Could you check a few things on this model? Use its own coordinates, in mm. A direction names the side the tool comes from. Coordinates: 2 decimals unless noted, no trailing zeros. Loops run counter-clockwise (first coordinate to the right, second up) from the corner with the lowest first, then second, coordinate; pieces in that order, holes last. Notation, with made-up numbers: (41.25, -9) - (50.25, -9) arc R14 ccw to (50.25, 15) - close; hole circle Ø2 at (4, 9.5). An arc over 180 degrees is marked (long way). Put each result on its own line as item: value. Start each with the question number.
```python
from build123d import *

# Parameters (mm, degrees)
F1_DEPTH    = 25
F2_SIZE2    = 24.99999
F2_SIZE     = 77.78174
F4_DEPTH    = 130
F5_W        = 126.5929291126
F5_H        = 5
F6_DEPTH    = 25
F7_T1_DEPTH = 126.5929291126
F9_DEPTH    = 15


# Not quite as in the source:
# - a fillet or chamfer that OpenCascade refuses, or shapes differently, is made with other operations: its cross-section is extruded or revolved along the edge and cut away or added
# - a fillet or chamfer is up to 0.001 mm smaller than in the source, because OpenCascade refuses the exact size


with BuildPart() as f1:
    # F0 (on Top) → F1 (new body)
    with BuildSketch(Plane.XY):
        Polygon((55, 55), (-55, 55), (-55, -55), align=None)
    extrude(amount=F1_DEPTH)

    # F2 (size 77.78175 and 25 in the source; OpenCascade refuses exactly that, so slightly less here)
    f2_edges = [f1.edges().sort_by_distance(p)[0] for p in [
        (0, 0, 25),
    ]]
    f2_side = f1.faces().sort_by_distance((-18.333333, 18.333333, 25))[0]
    chamfer(f2_edges, length=F2_SIZE, length2=F2_SIZE2, reference=f2_side)

    # F3 (on Top) → F4 (join)
    with BuildSketch(Plane.XY):
        Polygon((-55, 55), (-55, -55), (55, 55), align=None)
        Polygon((-49, -40.5147186258), (-49, 49), (40.5147186258, 49), align=None, mode=Mode.SUBTRACT)
    extrude(amount=F4_DEPTH)

    # F5 (on face) → F6 (cut)
    with BuildSketch(Plane(origin=(-4.2426406871, 4.2426406871, 0), x_dir=(-0.7071067812, -0.7071067812, 0), z_dir=(-0.7071067812, 0.7071067812, 0))):
        with Locations((0, 4.4284729387)):
            Rectangle(F5_W, F5_H)
    extrude(amount=-F6_DEPTH, mode=Mode.SUBTRACT)

    # F7: chamfer of 6 x 2 on 1 edges, made by hand

    # F7_s2 → F7_t1 (cut)
    with BuildSketch(Plane(origin=(44.7573593129, 44.7573593129, 0), x_dir=(0, 0, 1), z_dir=(-0.7071067812, -0.7071067812, 0))):
        Polygon((-0.0715270613, 0), (1.9284729387, 6), (1.9284729387, 0), align=None)
    extrude(amount=F7_T1_DEPTH, mode=Mode.SUBTRACT)

    # F8 (on face) → F9 (join)
    with BuildSketch(Plane.XY.offset(130)):
        Polygon((-45.4644660941, 49), (-49, 49), (-49, 45.4644660941), (-35.8485209767, 32.3129870708), (-49, 19.1615080475), (-49, 14.1615080475), (-42.9420274413, 20.2194806062), (-36.7324044532, 1.5906116418), (-49, -10.676983905), (-49, -15.676983905), (-35.4824044532, -2.1593883582), (-29.272970773, -20.7876893988), (-25.7374368671, -17.2521554928), (-31.9468705473, 1.3761455477), (-18.4292750005, 14.8937410945), (-6.0104076401, 2.4748737342), (-4.2426406871, 4.2426406871), (-2.4748737342, 6.0104076401), (-14.8937410945, 18.4292750005), (-1.3761455477, 31.9468705473), (17.2521554928, 25.7374368671), (20.7876893988, 29.272970773), (2.1593883582, 35.4824044532), (15.676983905, 49), (10.676983905, 49), (-1.5906116418, 36.7324044532), (-20.2194806062, 42.9420274413), (-14.1615080475, 49), (-19.1615080475, 49), (-32.3129870708, 35.8485209767), align=None)
        Polygon((-33.3485209767, 29.8129870708), (-20.9292750005, 17.3937410945), (-33.1968705473, 5.1261455477), (-39.4064935354, 23.7550145121), align=None, mode=Mode.SUBTRACT)
        Polygon((-17.3937410945, 20.9292750005), (-29.8129870708, 33.3485209767), (-23.7550145121, 39.4064935354), (-5.1261455477, 33.1968705473), align=None, mode=Mode.SUBTRACT)
    extrude(amount=-F9_DEPTH)


solid = f1.part
```
(1) If we mould it in two halves opening along X, with no side actions, what happens to faces 4 (the flat face through (-1, -1, 64)), 5 (the flat face through (1, 55, 64)), 6 (the flat face through (-42.336, -9.013, 122.605))? For each: pulls with the +X half, pulls with the -X half, needs draft (parallel to the pull), parting line crosses it, or undercut.
(2) I need wall thicknesses on L1, parallel to X at y = -14, z = 119; L2, parallel to Y at x = 25, z = 123.5; L3, parallel to Y at x = -9, z = 112.5. Which ranges of each line are inside material? Lowest first, please. Write a range as [from, to].
(3) I want a section at C-C on x = 5.5. Count the separate pieces of the cut face and the enclosed holes in it, and give its area (3 significant figures).
(4) For pin 1 Ø8 at (x, y) = (3, 20) entering from +Z; pin 2 Ø6 at (y, z) = (-23.5, 82.5) entering from +X, each with a flat end and sliding along its axis, tell me the tip position at first contact or that it passes through.
(5) I want a section at B-B on z = 80.5. List the corners of the cut face in (x, y) for me, and give its area (3 significant figures).
(6) Which directions (+Z, -Z, +X, -X, +Y, -Y) give clear straight access to the entire face, cutting with the end or side of a thin tool? Please do faces 1 (the flat face through (42.606, 46.908, 4.283)), 2 (the flat face through (-36.26, 14.31, 122.6)), 3 (the flat face through (-46.908, -42.606, 4.283)).
Answer sheet:
1. face 4: pulls with the +X half
1. face 5: needs draft
1. face 6: undercut
2. L1: x = [-55, -47.32], [-31.54, -26.82], [-22.49, -14]
2. L2: y = [25, 33.49], [49, 55]
2. L3: y = [-9, -0.51], [49, 55]
3. separate pieces: 4
3. enclosed holes: 0
3. area: 2,180 mm^2
4. pin 1: stops at z = 5.15
4. pin 2: stops at x = -20.5
5. outline: (-55, -55) - (55, 55) - (-55, 55) - close; hole (-49, -40.51) - (40.51, 49) - (-49, 49) - close
5. area: 2,040 mm^2
6. face 1: -Y
6. face 2: +Z
6. face 3: +X
